Check sheet for the modelled part. Datum: model origin and axes. Units: mm. Face numbers are marked on the shaded views. Coordinates: 2 decimals unless noted, no trailing zeros. Order: outer loops, then holes, each group sorted by start corner. A loop starts at its lowest first (then second) coordinate and runs counter-clockwise, first axis right, second up. Notation, with made-up numbers: M -13.75,-5 L -0.75,-5 A20 cw -0.75,-1 Z; hole C 59.5,56 d10. An arc over 180 degrees is marked long. Answer in a Markdown table with one row per item. Add a question column.
from build123d import *

# Parameters (mm, degrees)
BOSS_EXTRUDE3_DEPTH = 1.25
SKETCH5_R           = 1.45
CUT_EXTRUDE1_DEPTH  = 1.25
SKETCH6_R           = 8
BOSS_EXTRUDE6_DEPTH = 20
SKETCH8_R           = 6
CUT_EXTRUDE5_DEPTH  = 30
SKETCH9_R           = 7
CUT_EXTRUDE7_DEPTH  = 25
SKETCH10_R          = 52.083932338
CUT_EXTRUDE9_DEPTH  = 0.25
SKETCH11_W          = 15
SKETCH11_H          = 15
BOSS_EXTRUDE9_DEPTH = 1


with BuildPart() as part:
    # Sketch1 → Boss-Extrude3 (new body)
    with BuildSketch(Plane(origin=(0, 0, 0), x_dir=(1, 0, 0), z_dir=(0, 1, 0))):
        Polygon((0, 50), (43.301270189, -25), (0, 0), align=None)
        Polygon((0, 0), (0, 50), (-43.301270189, -25), align=None)
        Polygon((0, 0), (-43.301270189, -25), (43.301270189, -25), align=None)
    extrude(amount=BOSS_EXTRUDE3_DEPTH)

    # Sketch5 → Cut-Extrude1 (cut)
    with BuildSketch(Plane(origin=(0, 1.25, 0), x_dir=(1, 0, 0), z_dir=(0, 1, 0))):
        with Locations(Location((0, 37.25, 0), (0, 0, 270))):
            Circle(SKETCH5_R)
        with Locations(Location((-32.259446291, -18.625, 0), (0, 0, 270))):
            Circle(SKETCH5_R)
        with Locations(Location((32.259446291, -18.625, 0), (0, 0, 270))):
            Circle(SKETCH5_R)
    extrude(amount=-CUT_EXTRUDE1_DEPTH, mode=Mode.SUBTRACT)

    # Sketch6 → Boss-Extrude6 (add)
    with BuildSketch(Plane.XZ):
        with Locations(Location((0, 0, 0), (0, 0, 90))):
            Circle(SKETCH6_R)
    extrude(amount=BOSS_EXTRUDE6_DEPTH)

    # Sketch8 → Cut-Extrude5 (cut)
    with BuildSketch(Plane.XZ.offset(20)):
        with Locations(Location((0, 0, 0), (0, 0, 270))):
            Circle(SKETCH8_R)
    extrude(amount=-CUT_EXTRUDE5_DEPTH, mode=Mode.SUBTRACT)

    # Sketch9 → Cut-Extrude7 (cut)
    with BuildSketch(Plane.XZ.offset(20)):
        with Locations(Location((0, 0, 0), (0, 0, 270))):
            Circle(SKETCH9_R)
    extrude(amount=-CUT_EXTRUDE7_DEPTH, mode=Mode.SUBTRACT)

    # Sketch10 → Cut-Extrude9 (cut)
    with BuildSketch(Plane(origin=(0, 1.25, 0), x_dir=(1, 0, 0), z_dir=(0, 1, 0))):
        Circle(SKETCH10_R)
    extrude(amount=-CUT_EXTRUDE9_DEPTH, mode=Mode.SUBTRACT)

    # Sketch11 → Boss-Extrude9 (add)
    with BuildSketch(Plane.XZ):
        with Locations((0, -50)):
            Rectangle(SKETCH11_W, SKETCH11_H)
    extrude(amount=-BOSS_EXTRUDE9_DEPTH)


solid = part.part
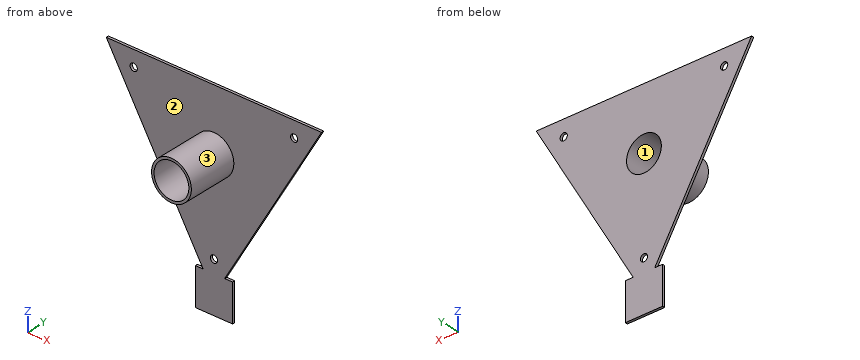
1. Go/stop test with flat-tipped pins: pin 1 Ø12 at (x, z) = (25, -30.5) entering from +Y; pin 2 Ø12 at (x, z) = (21, 6.5) entering from -Y; pin 3 Ø2 at (x, y) = (-5, -1.5) entering from +Z; pin 4 Ø0.8 at (y, z) = (0.5, -52.5) entering from -X. Record where each tip stops, or that it passes through.
2. Section check C-C on y = -14. Enter the section's corners in (x, z), then the cut area to 3 significant figures.
3. Scan lines: line 1 (X direction, y = -1, z = 0); line 2 (Y direction, x = 28, z = 3); line 3 (Z direction, x = -3.5, y = -10.5). Record each from-to range of solid material in increasing order.
4. Section check A-A on x = 0. Enter the section's corners in (y, z), then the cut area to 3 significant figures.
5. Section check D-D on z = 0. Enter the section's corners in (x, y).
6. Section check B-B on z = -37.25. Enter the section's corners in (x, y), then the cut area to 3 significant figures.
7. Release check for a two-part mould opening along Z. For the marked faces 1, 2 and 3 record: released by +Z, released by -Z, zero draft, split by the parting line, or undercut.
Result sheet:
| question | item | result |
|---|---|---|
| 1 | pin 1 | through |
| 1 | pin 2 | y = 0 |
| 1 | pin 3 | z = 6.93 |
| 1 | pin 4 | x = -7.5 |
| 2 | outline | C 0,0 d16; hole C 0,0 d14 |
| 2 | area | 47.1 mm^2 |
| 3 | line 1 | -8 to -7, 7 to 8 |
| 3 | line 2 | 0 to 1 |
| 3 | line 3 | -7.19 to -6.06, 6.06 to 7.19 |
| 4 | outline | M -20,-8 L 0,-8 L 0,-35.8 L 1,-35.8 L 1,-7 L -20,-7 Z; M -20,7 L 1,7 L 1,25 L 0,25 L 0,8 L -20,8 Z; M 0,-57.5 L 1,-57.5 L 1,-38.7 L 0,-38.7 Z |
| 4 | area | 106 mm^2 |
| 5 | outline | M -28.87,0 L -8,0 L -8,-20 L -7,-20 L -7,1 L -28.87,1 Z; M 7,-20 L 8,-20 L 8,0 L 28.87,0 L 28.87,1 L 7,1 Z |
| 6 | outline | M -7.36,0 L -1.45,0 L -1.45,1 L -7.36,1 Z; M 1.45,0 L 7.36,0 L 7.36,1 L 1.45,1 Z |
| 6 | area | 11.8 mm^2 |
| 7 | face 1 | undercut |
| 7 | face 2 | zero draft |
| 7 | face 3 | split by the parting line |
